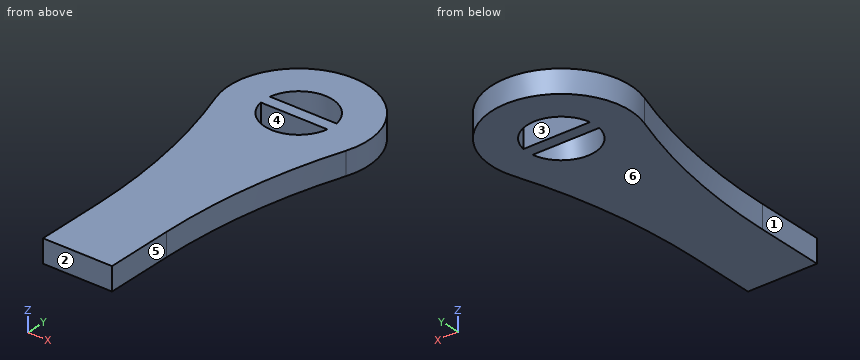
```python
from build123d import *

# Parameters (mm, degrees)
BOSS_EXTRUDE1_DEPTH = 2


with BuildPart() as part:
    # Model → Boss-Extrude1 (new body)
    with BuildSketch(Plane.XY):
        with BuildLine():
            Line((58.08314132, -82), (58.08314132, -87.91685868))
            Line((58.08314132, -87.91685868), (52.08314132, -87.91685868))
            Line((52.08314132, -87.91685868), (52.08314132, -82))
            ThreePointArc((52.08314132, -82), (51.408953166, -73.816829116), (49.404569891, -65.854338107))
            ThreePointArc((49.404569891, -65.854338107), (55.08314132, -57.91685868), (60.761712749, -65.854338107))
            ThreePointArc((60.761712749, -65.854338107), (58.757329474, -73.816829116), (58.08314132, -82))
        make_face()
        with BuildLine():
            Line((52.188507276, -64.41685868), (57.977775364, -64.41685868))
            ThreePointArc((57.977775364, -64.41685868), (55.08314132, -66.85435868), (52.188507276, -64.41685868))
        make_face(mode=Mode.SUBTRACT)
        with BuildLine():
            Line((57.977775364, -63.41685868), (52.188507276, -63.41685868))
            ThreePointArc((52.188507276, -63.41685868), (55.08314132, -60.97935868), (57.977775364, -63.41685868))
        make_face(mode=Mode.SUBTRACT)
    extrude(amount=BOSS_EXTRUDE1_DEPTH)


solid = part.part
```
Design review of the part built by this model. Coordinates are the model's own, in mm. Face numbers are marked on the shaded views. A direction names the side the tool comes from. Give positions to 0.01 mm unless a question says otherwise; leave off trailing zeros. Write each loop counter-clockwise with the first axis right and the second up, starting at its lowest first coordinate (ties: lowest second). Pieces come first, ordered by that corner, then holes. Notation, with made-up numbers: (20.25, -11) - (32.25, -11) arc R32 cw to (32.25, 28) - close; hole circle Ø4 at (33, 3). An arc over 180 degrees is marked (long way). Return JSON: item names as keys, results as strings. Group by question number.
(1) We need section D-D, the plane x = 56.75. Give the boundary of the cut face in (y, z).
(2) Mouldability with a two-part tool opening along Y and no side actions: class the marked faces 1, 2 and 3 as +Y half, -Y half, draft (parallel to the pull), parting line (faces both ways), or undercut.
(3) We need section B-B, the plane x = 53.5. Give the boundary of the cut face in (y, z), then the cut area to 3 significant figures.
(4) Insertion check: pin 1 (1 mm diameter, centred on y = -86, z = 0.5, fed in from +X). The pin has a flat end and moves straight along its axis. Give the tip position at first contact, or say it passes through.
(5) We need section A-A, the plane z = 0.95. Give the boundary of the cut face in (x, y) (1 decimal), then the cut area to 3 significant figures.
(6) We need section C-C, the plane y = -80.5. Give the boundary of the cut face in (x, z).
(7) To check wall thickness, follow probe 1 along Y at (x, z) = (55, 0.8); probe 2 along Y at (x, z) = (57, 1); probe 3 along X at (y, z) = (-86, 1). State the ranges of each line that lie inside material, in increasing order.
(8) Machinability: for the marked faces 4, 5 and 6, which of the approach directions +Z, -Z, +X, -X, +Y, -Y give a long, thin tool a straight path to every point of the face, cutting with its end or side? Answer none if there is none.
Reported:
{
 "1": {"outline": "(-87.92, 0) - (-66.34, 0) - (-66.34, 2) - (-87.92, 2) - close; (-64.42, 0) - (-63.42, 0) - (-63.42, 2) - (-64.42, 2) - close; (-61.5, 0) - (-58.15, 0) - (-58.15, 2) - (-61.5, 2) - close"},
 "2": {"face 1": "draft", "face 2": "-Y half", "face 3": "undercut"},
 "3": {"outline": "(-87.92, 0) - (-66.39, 0) - (-66.39, 2) - (-87.92, 2) - close; (-64.42, 0) - (-63.42, 0) - (-63.42, 2) - (-64.42, 2) - close; (-61.44, 0) - (-58.13, 0) - (-58.13, 2) - (-61.44, 2) - close", "area": "51.7 mm2"},
 "4": {"pin 1": "stops at x = 58.08"},
 "5": {"outline": "(49.4, -65.9) arc R50 cw to (52.1, -82) - (52.1, -87.9) - (58.1, -87.9) - (58.1, -82) arc R50 cw to (60.8, -65.9) arc R6 ccw (long way) to start; hole (52.2, -64.4) arc R2.9 ccw to (58, -64.4) - close; hole (52.2, -63.4) - (58, -63.4) arc R2.9 ccw to start", "area": "219 mm2"},
 "6": {"outline": "(52.06, 0) - (58.11, 0) - (58.11, 2) - (52.06, 2) - close"},
 "7": {"probe 1": "y = -87.92 to -66.85, -64.42 to -63.42, -60.98 to -57.92", "probe 2": "y = -87.92 to -66.14, -64.42 to -63.42, -61.69 to -58.23", "probe 3": "x = 52.08 to 58.08"},
 "8": {"face 4": "+Z, -Z", "face 5": "+Z, -Z, +X, -Y", "face 6": "-Z, +X, -X, +Y, -Y"}
}
